Can you work these out from the model? Positions are in its coordinate system, mm. Face numbers are marked on the shaded views. Give positions to 0.01 mm unless a question says otherwise; leave off trailing zeros. Loops run counter-clockwise (first coordinate to the right, second up) from the corner with the lowest first, then second, coordinate; pieces in that order, holes last. Notation, with made-up numbers: (19, 55.25) - (49, 55.25) arc R24 cw to (49, 92.25) - close; hole circle Ø6 at (-31.75, 2.5). An arc over 180 degrees is marked (long way). Answer as a JSON object with one key per item and string values.
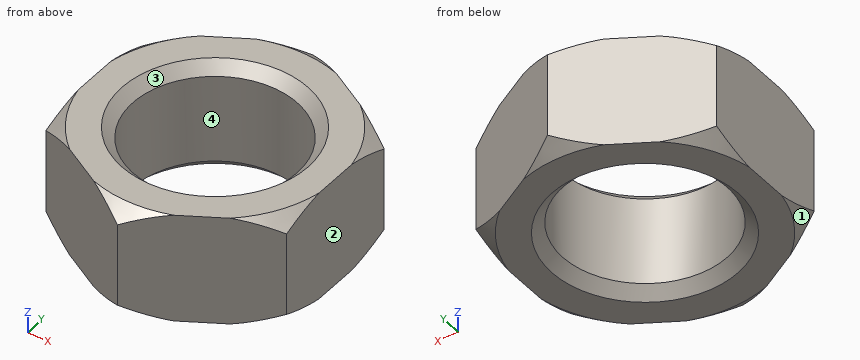
```python
from build123d import *

# Parameters (mm, degrees)
BOSS_EXTRUDE1_DEPTH = 10
SKETCH2_R           = 7.5
CUT_EXTRUDE1_DEPTH  = 20.553345835
CHAMFER1_SIZE       = 1
SCALE1_SCALE        = 0.25


with BuildPart() as part:
    # Sketch1 → Boss-Extrude1 (new body)
    with BuildSketch(Plane.XY):
        Polygon((11, -6.350852961), (11, 6.350852961), (0, 12.701705922), (-11, 6.350852961), (-11, -6.350852961), (0, -12.701705922), align=None)
    extrude(amount=BOSS_EXTRUDE1_DEPTH)

    # Sketch2 → Cut-Extrude1 (cut, through all)
    with BuildSketch(Plane.XY.offset(10)):
        Circle(SKETCH2_R)
    extrude(amount=-CUT_EXTRUDE1_DEPTH, mode=Mode.SUBTRACT)

    # Chamfer1
    chamfer1_edges = [part.edges().sort_by_distance(p)[0] for p in [
        (-7.5, 0, 0),
        (-7.5, 0, 10),
    ]]
    chamfer(chamfer1_edges, length=CHAMFER1_SIZE)

    # Sketch3 → Cut-Revolve1 (revolve, cut)
    with BuildSketch(Plane(origin=(0, 0, 0), x_dir=(0, 0, -1), z_dir=(1, 0, 0))):
        Polygon((-1.2, 12.701705922), (0, 11.201705922), (0, 12.701705922), align=None)
        Polygon((-10, 12.701705922), (-8.8, 12.701705922), (-10, 11.201705922), align=None)
    revolve(axis=Axis((0, 0, 11.931006721), (0, 0, -1)), mode=Mode.SUBTRACT)


with BuildPart() as part_1:
    # Scale1: scaled about (0, 0, 5)
    add(part.part.scale(SCALE1_SCALE).moved(Location((0, 0, 3.75))))


solid = part_1.part
```
1) Imagine slicing it at B-B on z = 4.15. Write out the boundary of the cut face in (x, y) (3 decimals).
Check sheet entries:
{"outline": "(-2.75, -1.588) - (0, -3.175) - (2.75, -1.588) - (2.75, 1.588) - (0, 3.175) - (-2.75, 1.588) - close; hole circle Ø3.75 at (0, 0)"}
2) Imagine slicing it at A-A on y = 0. Write out the boundary of the cut face in (x, z) (3 decimals).
Check sheet entries:
{"outline": "(-2.75, 3.75) - (-2.125, 3.75) - (-1.875, 4) - (-1.875, 6) - (-2.125, 6.25) - (-2.75, 6.25) - close; (1.875, 4) - (2.125, 3.75) - (2.75, 3.75) - (2.75, 6.25) - (2.125, 6.25) - (1.875, 6) - close"}
3) If we mould it in two halves opening along X, with no side actions, what happens to the marked faces 1, 2, 3 and 4? For each: released by +X, released by -X, zero draft, split by the parting line, or undercut.
Check sheet entries:
{"face 1": "released by -X", "face 2": "released by +X", "face 3": "undercut", "face 4": "undercut"}
4) I need wall thicknesses on L1, parallel to X at y = -1, z = 5.05; L2, parallel to Y at x = 0.6, z = 5.6; L3, parallel to X at y = 0.75, z = 5.9. Which ranges of each line are inside material? Lowest first, please.
Check sheet entries:
{"L1": "-2.75 to -1.59, 1.59 to 2.75", "L2": "-2.83 to -1.78, 1.78 to 2.83", "L3": "-2.75 to -1.72, 1.72 to 2.75"}
